The model under review builds one solid part; all positions refer to its coordinate system, in mm. A direction names the side the tool comes from. Coordinates: 2 decimals unless noted, no trailing zeros. Loops run counter-clockwise (first coordinate to the right, second up) from the corner with the lowest first, then second, coordinate; pieces in that order, holes last. Notation, with made-up numbers: M 43.5,-39 L 66.5,-39 A25 cw 66.5,-22 Z; hole C -38.75,59.25 d10. An arc over 180 degrees is marked long. One line per item, written item: value.
```python
from build123d import *

# Parameters (mm, degrees)
SKETCH_W        = 41.2
SKETCH_H        = 41.2
PAD_DEPTH       = 45.2
SKETCH001_R     = 11
PAD001_DEPTH    = 47.2
SKETCH002_R     = 11.1
POCKET_DEPTH    = 38.7
SKETCH003_W     = 35.7
SKETCH003_H     = 35.7
POCKET001_DEPTH = 36.7
SKETCH004_R     = 1.5
SKETCH004_R_2   = 1.25
POCKET002_DEPTH = 45.201
SKETCH005_R     = 3.75
POCKET003_DEPTH = 4
SKETCH006_R     = 6
POCKET004_DEPTH = 47.201
SKETCH007_W     = 55
SKETCH007_H     = 5
POCKET005_DEPTH = 12
CHAMFER_SIZE    = 2
SKETCH008_W     = 9
SKETCH008_H     = 9
PAD002_DEPTH    = 3
SKETCH009_R     = 1.75
POCKET006_DEPTH = 47.201
CHAMFER001_SIZE = 1.75


with BuildPart() as part:
    # Sketch → Pad (new body)
    with BuildSketch(Plane.XY):
        Rectangle(SKETCH_W, SKETCH_H)
    extrude(amount=PAD_DEPTH)

    # Sketch001 → Pad001 (join)
    with BuildSketch(Plane.XY):
        Circle(SKETCH001_R)
    extrude(amount=PAD001_DEPTH)

    # Sketch002 → Pocket (cut)
    with BuildSketch(Plane.XY):
        Circle(SKETCH002_R)
    extrude(amount=POCKET_DEPTH, mode=Mode.SUBTRACT)

    # Sketch003 → Pocket001 (cut)
    with BuildSketch(Plane.XY):
        Rectangle(SKETCH003_W, SKETCH003_H)
    extrude(amount=POCKET001_DEPTH, mode=Mode.SUBTRACT)

    # Sketch004 (on DatumPlane) → Pocket002 (cut, through all)
    with BuildSketch(Plane.XY.offset(45.2)):
        with Locations((13, 13)):
            Circle(SKETCH004_R)
        with Locations((15.5, 0)):
            Circle(SKETCH004_R_2)
        with Locations((-13, 13)):
            Circle(SKETCH004_R)
        with Locations((0, 15.5)):
            Circle(SKETCH004_R_2)
        with Locations((-15.5, 0)):
            Circle(SKETCH004_R_2)
        with Locations((0, -15.5)):
            Circle(SKETCH004_R_2)
        with Locations((13, -13)):
            Circle(SKETCH004_R)
        with Locations((-13, -13)):
            Circle(SKETCH004_R)
    extrude(amount=-POCKET002_DEPTH, mode=Mode.SUBTRACT)

    # Sketch005 (on DatumPlane) → Pocket003 (cut)
    with BuildSketch(Plane.XY.offset(45.2)):
        with Locations((-13, 13)):
            Circle(SKETCH005_R)
        with Locations((13, 13)):
            Circle(SKETCH005_R)
        with Locations((13, -13)):
            Circle(SKETCH005_R)
        with Locations((-13, -13)):
            Circle(SKETCH005_R)
    extrude(amount=-POCKET003_DEPTH, mode=Mode.SUBTRACT)

    # Sketch006 → Pocket004 (cut, through all)
    with BuildSketch(Plane.XY):
        Circle(SKETCH006_R)
    extrude(amount=POCKET004_DEPTH, mode=Mode.SUBTRACT)

    # Sketch007 → Pocket005 (cut)
    with BuildSketch(Plane.XY):
        Rectangle(SKETCH007_W, SKETCH007_H)
    extrude(amount=POCKET005_DEPTH, mode=Mode.SUBTRACT)

    # Chamfer
    chamfer_edges = [part.edges().sort_by_distance(p)[0] for p in [
        (19.225, 2.5, 12),
        (19.225, -2.5, 12),
        (-19.225, -2.5, 12),
        (-19.225, 2.5, 12),
    ]]
    chamfer(chamfer_edges, length=CHAMFER_SIZE)

    # Sketch008 → Pad002 (join)
    with BuildSketch(Plane.XY):
        with Locations((-25.1, 16.1)):
            Rectangle(SKETCH008_W, SKETCH008_H)
        with Locations((25.1, 16.1)):
            Rectangle(SKETCH008_W, SKETCH008_H)
        with Locations((25.1, -16.1)):
            Rectangle(SKETCH008_W, SKETCH008_H)
        with Locations((-25.1, -16.1)):
            Rectangle(SKETCH008_W, SKETCH008_H)
    extrude(amount=PAD002_DEPTH)

    # Sketch009 → Pocket006 (cut, through all)
    with BuildSketch(Plane.XY):
        with Locations((-25.1, 16.1)):
            Circle(SKETCH009_R)
        with Locations((-25.1, -16.1)):
            Circle(SKETCH009_R)
        with Locations((25.1, -16.1)):
            Circle(SKETCH009_R)
        with Locations((25.1, 16.1)):
            Circle(SKETCH009_R)
    extrude(amount=POCKET006_DEPTH, mode=Mode.SUBTRACT)

    # Chamfer001
    chamfer001_edges = [part.edges().sort_by_distance(p)[0] for p in [
        (-26.85, 16.1, 3),
        (-26.85, -16.1, 3),
        (23.35, 16.1, 3),
        (23.35, -16.1, 3),
    ]]
    chamfer(chamfer001_edges, length=CHAMFER001_SIZE)


solid = part.part
```
(1) Add section B-B on x = 0. State the section outline as (y, z) points, then the cut area to 3 significant figures.
Checks:
outline: M -20.6,0 L -17.85,0 L -17.85,36.7 L -16.75,36.7 L -16.75,45.2 L -20.6,45.2 Z; M -14.25,36.7 L -11.1,36.7 L -11.1,38.7 L -6,38.7 L -6,47.2 L -11,47.2 L -11,45.2 L -14.25,45.2 Z; M 6,38.7 L 11.1,38.7 L 11.1,36.7 L 14.25,36.7 L 14.25,45.2 L 11,45.2 L 11,47.2 L 6,47.2 Z; M 16.75,36.7 L 17.85,36.7 L 17.85,0 L 20.6,0 L 20.6,45.2 L 16.75,45.2 Z
area: 407 mm^2
(2) To check wall thickness, follow L1, parallel to Y at x = 0, z = 38.35; L2, parallel to Y at x = 13, z = 38; L3, parallel to Y at x = 16.5, z = 12. State the ranges of each line that lie inside material, in increasing order. Write a range as [from, to].
Checks:
L1: [-20.6, -16.75], [-14.25, -11.1], [11.1, 14.25], [16.75, 20.6]
L2: [-20.6, -14.5], [-11.5, 11.5], [14.5, 20.6]
L3: [-20.6, -17.85], [17.85, 20.6]
(3) Add section C-C on z = 7. State the section outline as (x, y) points.
Checks:
outline: M -20.6,-20.6 L 20.6,-20.6 L 20.6,-2.5 L 17.85,-2.5 L 17.85,-17.85 L -17.85,-17.85 L -17.85,-2.5 L -20.6,-2.5 Z; M -20.6,2.5 L -17.85,2.5 L -17.85,17.85 L 17.85,17.85 L 17.85,2.5 L 20.6,2.5 L 20.6,20.6 L -20.6,20.6 Z
(4) Add section A-A on x = -13. State the section outline as (y, z) points, then the cut area to 3 significant figures.
Checks:
outline: M -20.6,0 L -17.85,0 L -17.85,36.7 L -14.5,36.7 L -14.5,41.2 L -16.75,41.2 L -16.75,45.2 L -20.6,45.2 Z; M -11.5,36.7 L 11.5,36.7 L 11.5,41.2 L 9.25,41.2 L 9.25,45.2 L -9.25,45.2 L -9.25,41.2 L -11.5,41.2 Z; M 14.5,36.7 L 17.85,36.7 L 17.85,0 L 20.6,0 L 20.6,45.2 L 16.75,45.2 L 16.75,41.2 L 14.5,41.2 Z
area: 465 mm^2
(5) Insertion check: pin 1 Ø2.5 at (x, y) = (-13, -13) entering from -Z; pin 2 Ø5 at (y, z) = (8.5, 33) entering from +X; pin 3 Ø5 at (x, y) = (-4.5, 10) entering from -Z; pin 4 Ø6 at (x, y) = (-13, 13) entering from +Z. Each pin has a flat end and moves straight along its axis. Give the tip position at first contact, or say it passes through.
Checks:
pin 1: through
pin 2: x = 20.6
pin 3: z = 36.7
pin 4: z = 41.2
(6) Tool access review of faces 1 (the face through (-28.2, 18.2, 3)), 2 (the face through (-15.764, 15.534, 43.228)), 3 (the face through (-25, -11.6, 1)): name each direction out of +Z, -Z, +X, -X, +Y, -Y from which nothing blocks a thin tool from reaching the whole face with its end or side.
Checks:
face 1: +Z, -X, +Y, -Y
face 2: +Z
face 3: +Z, -Z, -X
(7) Add section D-D on z = 37.5. State how many separate pieces and enclosed holes the cut face has, then the cut area to 3 significant figures.
Checks:
separate pieces: 1
enclosed holes: 9
area: 1,260 mm^2
